Source: CAD feature listing. Evaluate the final solid. Frame: model axes, mm. Coordinates: 2 decimals unless noted, no trailing zeros. Order: outer loops, then holes, each group sorted by start corner. A loop starts at its lowest first (then second) coordinate and runs counter-clockwise, first axis right, second up. Notation, with made-up numbers: (60, 48.25) - (92, 48.25) arc R7 ccw to (92, 57.25) - close; hole circle Ø4 at (82, -19). An arc over 180 degrees is marked (long way). One line per question, with ' | ' between items.
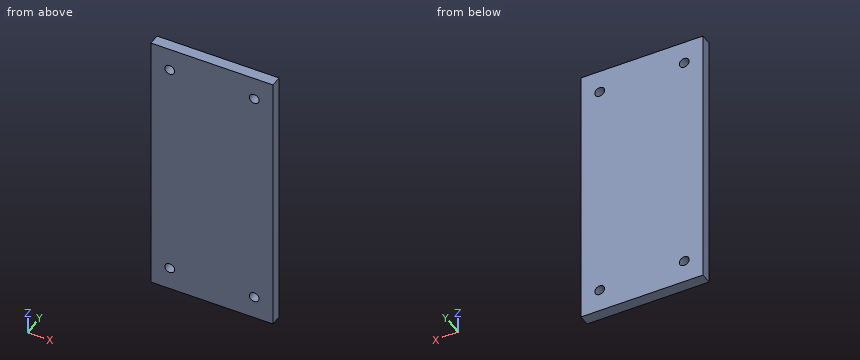
Autodesk Inventor part; units mm, degrees
ref_plane "YZ Plane" through (0, 0, 0) normal (1, 0, 0) x (0, 1, 0)
ref_plane "XZ Plane" through (0, 0, 0) normal (0, 1, 0) x (-1, 0, 0)
ref_plane "XY Plane" through (0, 0, 0) normal (0, 0, 1) x (1, 0, 0)
sketch "Sketch1" plane through (0, 0, 0) normal (0, 1, 0) x (-1, 0, 0)
  line L0 (0, 0) -> (22, 0)
  line L1 (22, 0) -> (22, -49)
  line L2 (22, -49) -> (0, -49)
  line L3 (0, -49) -> (0, 0)
  dimension "d0" = 22
  dimension "d1" = 49
extrude "Extrusion1" add sketch "Sketch1" along normal blind 2
sketch "Sketch2" plane through (0, 2, 0) normal (0, 1, 0) x (1, 0, 0)
  line L0 (-22, 0) -> (0, 0)
  line L1 (0, 0) -> (0, 49)
  line L2 (-18.62, 44.82) -> (-3.38, 44.82) construction
  line L3 (-3.38, 44.82) -> (-3.38, 4.18) construction
  line L4 (-3.38, 4.18) -> (-18.62, 4.18) construction
  line L5 (-18.62, 4.18) -> (-18.62, 44.82) construction
  line L6 (-18.62, 44.82) -> (-3.38, 4.18) construction
  line L7 (-3.38, 44.82) -> (-18.62, 4.18) construction
  circle A0 centre (-18.62, 4.18) radius 0.885
  circle A1 centre (-18.62, 44.82) radius 0.885
  circle A2 centre (-3.38, 44.82) radius 0.885
  circle A3 centre (-3.38, 4.18) radius 0.885
  point P0 (0, 24.5)
  point P1 (-11, 0)
  point P2 (-3.38, 0)
  point P3 (0, 4.18)
  point P4 (-11, 24.5)
  dimension "d4" = 11
  dimension "d5" = 7.62
  dimension "d6" = 20.32
  dimension "d8" = 1.77
  dimension "d9" = 1.77
  dimension "d10" = 1.77
  dimension "d11" = 1.77
extrude "Extrusion2" cut sketch "Sketch2" against normal up to next
properties part number "plate4atrduino"
(1) Cut plane B-B (z = -4.18). Return the cut outline in (x, y) (3 decimals), and give its area (3 significant figures).
Taken from the geometry:
outline: (-22, 0) - (-19.505, 0) - (-19.505, 2) - (-22, 2) - close; (-17.735, 0) - (-4.265, 0) - (-4.265, 2) - (-17.735, 2) - close; (-2.495, 0) - (0, 0) - (0, 2) - (-2.495, 2) - close | area: 36.9 mm²
(2) Material intervals for L1, parallel to Z at x = -18.62, y = 0.9 (3 decimals); L2, parallel to X at y = 1.3, z = -44.82 (3 decimals), sorted ascending. Write a range as from..to.
Taken from the geometry:
L1: z = -49..-45.705, -43.935..-5.065, -3.295..0 | L2: x = -22..-19.505, -17.735..-4.265, -2.495..0
(3) Pin query (flat end, axial travel): P1, Ø1.4, axis at x = -3.38, z = -44.82, coming from the +Y side; P2, Ø3, axis at x = -8.5, z = -39.5, coming from the -Y side. Return the tip coordinate at first contact, or that it passes through.
Taken from the geometry:
P1: passes through | P2: stops at y = 0
(4) Cut plane A-A (x = -3.38). Return the cut outline in (y, z) (3 decimals).
Taken from the geometry:
outline: (0, -49) - (2, -49) - (2, -45.705) - (0, -45.705) - close; (0, -43.935) - (2, -43.935) - (2, -5.065) - (0, -5.065) - close; (0, -3.295) - (2, -3.295) - (2, 0) - (0, 0) - close
